from build123d import *

# Parameters (mm, degrees)
SKETCH1_R           = 6
BOSS_EXTRUDE1_DEPTH = 12
CUT_EXTRUDE1_REACH  = 80.064
SKETCH3_R           = 14


with BuildPart() as part:
    # Sketch1 → Boss-Extrude1 (new body)
    with BuildSketch(Plane(origin=(0, 0, 0), x_dir=(1, 0, 0), z_dir=(0, 1, 0))):
        with BuildLine():
            Line((-50.909090909, 17.699278596), (-12.727272727, 32.603934255))
            ThreePointArc((-12.727272727, 32.603934255), (0, 35), (12.727272727, 32.603934255))
            Line((12.727272727, 32.603934255), (50.909090909, 17.699278596))
            ThreePointArc((50.909090909, 17.699278596), (63, 0), (50.909090909, -17.699278596))
            Line((50.909090909, -17.699278596), (12.727272727, -32.603934255))
            ThreePointArc((12.727272727, -32.603934255), (0, -35), (-12.727272727, -32.603934255))
            Line((-12.727272727, -32.603934255), (-50.909090909, -17.699278596))
            ThreePointArc((-50.909090909, -17.699278596), (-63, 0), (-50.909090909, 17.699278596))
        make_face()
        with Locations(Location((-44, 0, 0), (0, 0, 270))):
            Circle(SKETCH1_R, mode=Mode.SUBTRACT)
        with Locations(Location((44, 0, 0), (0, 0, 270))):
            Circle(SKETCH1_R, mode=Mode.SUBTRACT)
    extrude(amount=BOSS_EXTRUDE1_DEPTH)

    # Sketch2 → Revolve1 (revolve)
    with BuildSketch(Plane.XY, mode=Mode.PRIVATE) as revolve1_sk:
        Polygon((-14, 33.917096231), (-14, 12), (-28, 12), (-28, 42), align=None)
    revolve(revolve1_sk.sketch.rotate(Axis((0, 0, 0), (0, 1, 0)), 270), axis=Axis((0, 0, 0), (0, 1, 0)))

    # Sketch3 → Cut-Extrude1 (cut, up to next)
    with BuildSketch(Plane(origin=(0, 12, 0), x_dir=(1, 0, 0), z_dir=(0, 1, 0)), mode=Mode.PRIVATE) as cut_extrude1_sk1:
        with Locations(Location((0, 0, 0), (0, 0, 90))):
            Circle(SKETCH3_R)
    cut_extrude1_tool1 = extrude(cut_extrude1_sk1.sketch, amount=-CUT_EXTRUDE1_REACH, mode=Mode.PRIVATE) & part.part
    add(cut_extrude1_tool1.solids().sort_by_distance((0, 12, 0))[0], mode=Mode.SUBTRACT)


solid = part.part
Work out the finished part from the listing and answer in its coordinate system (mm). A direction names the side the tool comes from. Give positions to 0.01 mm unless a question says otherwise; leave off trailing zeros. Loops run counter-clockwise (first coordinate to the right, second up) from the corner with the lowest first, then second, coordinate; pieces in that order, holes last. Notation, with made-up numbers: (-18, -9) -> (-6, -9) arc R25 ccw to (-6, 18) -> close; hole circle Ø5 at (30, 48). An arc over 180 degrees is marked (long way). Use a Markdown table: item, result. Add a question column.
1) Which of the six approach directions +Z, -Z, +X, -X, +Y, -Y give full straight-line access (tool end or side, diameter ignored) to faces 4 (the flat face through (-31.551, 5.916, 25.256)), 5 (the cylindrical face through (27.334, 27.21, 6.07))?
2) The part is cut by section C-C, the plane y = 20. Determine the outline of the cut face in (x, z).
3) Each of these flat-tipped pins is pushed along its axis until it touches: P1, Ø6, axis at y = 36.5, z = 3.5, coming from the -X side; P2, Ø1, axis at y = 10.5, z = -17, coming from the -X side; P3, Ø11, axis at x = -44, z = 0, coming from the +Y side; P4, Ø10, axis at x = 41.5, z = 7.5, coming from the +Y side. Where does it stop, or does it pass through?
4) The part is cut by section B-B, the plane x = 0. Determine the outline of the cut face in (y, z).
5) Consider line 1 along Y through (x, z) = (-25.5, 15.5); line 2 along X through (y, z) = (10, 12.5); line 3 along Y through (x, z) = (16, 17.5). Determine where each line is inside the solid, lowest interval first.
6) The part is cut by section A-A, the plane z = 0. Determine the outline of the cut face in (x, y), plus the area to 3 significant figures.
7) For a pull along X with two mould halves and no side action, classify faces 1 (the cylindrical face through (45.802, 5.916, 5.723)), 2 (the cylindrical face through (-63, 6, 0)), 3 (the flat face through (31.551, 5.916, -25.256)) as +X half, -X half, draft (parallel to the pull), parting line (faces both ways), or undercut.
8) The part is cut by section D-D, the plane x = -39.5. Determine the outline of the cut face in (y, z), plus the area to 3 significant figures.
Reported:
| question | item | result |
|---|---|---|
| 1 | face 4 | +Z, -X, +Y, -Y |
| 1 | face 5 | +Y |
| 2 | outline | circle Ø56 at (0, 0); hole circle Ø28 at (0, 0) |
| 3 | P1 | stops at x = -28 |
| 3 | P2 | stops at x = -53.42 |
| 3 | P3 | passes through |
| 3 | P4 | stops at y = 12 |
| 4 | outline | (0, -35) -> (12, -35) -> (12, -28) -> (42, -28) -> (33.92, -14) -> (0, -14) -> close; (0, 14) -> (33.92, 14) -> (42, 28) -> (12, 28) -> (12, 35) -> (0, 35) -> close |
| 5 | line 1 | y = 0 to 12 |
| 5 | line 2 | x = -58.31 to -6.3, 6.3 to 58.31 |
| 5 | line 3 | y = 0 to 39.52 |
| 6 | outline | (-63, 0) -> (-50, 0) -> (-50, 12) -> (-63, 12) -> close; (-38, 0) -> (-14, 0) -> (-14, 33.92) -> (-28, 42) -> (-28, 12) -> (-38, 12) -> close; (14, 0) -> (38, 0) -> (38, 12) -> (28, 12) -> (28, 42) -> (14, 33.92) -> close; (50, 0) -> (63, 0) -> (63, 12) -> (50, 12) -> close |
| 6 | area | 1,610 mm^2 |
| 7 | face 1 | undercut |
| 7 | face 2 | -X half |
| 7 | face 3 | +X half |
| 8 | outline | (0, -22.15) -> (12, -22.15) -> (12, -3.97) -> (0, -3.97) -> close; (0, 3.97) -> (12, 3.97) -> (12, 22.15) -> (0, 22.15) -> close |
| 8 | area | 436 mm^2 |
